from build123d import *

# Parameters (mm, degrees)
F0_W     = 150
F0_H     = 100
F1_DEPTH = 1.5
F2_R     = 1.5
F2_W     = 22.4
F2_H     = 12.1
F3_DEPTH = 3.001
F4_R     = 1.618849898
F4_R_2   = 1.6569654359
F4_R_3   = 1.6400542831
F4_R_4   = 1.6604885459
F5_DEPTH = 3.001


with BuildPart() as f1:
    # F0 (on Top) → F1 (new body, symmetric)
    with BuildSketch(Plane.XY):
        Rectangle(F0_W, F0_H)
    extrude(amount=F1_DEPTH, both=True)

    # F2 (on face) → F3 (cut, through all)
    with BuildSketch(Plane.XY.offset(1.5)):
        with Locations((-55, -30)):
            Circle(F2_R)
        with Locations((-27.3, -30)):
            Circle(F2_R)
        with Locations((-41.15, -30)):
            Rectangle(F2_W, F2_H)
        with Locations((27.3, -30)):
            Circle(F2_R)
        with Locations((55, -30)):
            Circle(F2_R)
        with Locations((41.15, -30)):
            Rectangle(F2_W, F2_H)
        with Locations((27.3, 30)):
            Circle(F2_R)
        with Locations((55, 30)):
            Circle(F2_R)
        with Locations((41.15, 30)):
            Rectangle(F2_W, F2_H)
        with Locations((-55, 30)):
            Circle(F2_R)
        with Locations((-27.3, 30)):
            Circle(F2_R)
        with Locations((-41.15, 30)):
            Rectangle(F2_W, F2_H)
    extrude(amount=-F3_DEPTH, mode=Mode.SUBTRACT)

    # F4 (on face) → F5 (cut, through all)
    with BuildSketch(Plane.XY.offset(1.5)):
        with Locations((-24.7324935626, 26.3731424032)):
            Circle(F4_R)
        with Locations((25.2215412911, 11.3385100679)):
            Circle(F4_R_2)
        with Locations((25.2285262104, -16.3567047299)):
            Circle(F4_R_3)
        with Locations((-25.7276298944, -21.3546585025)):
            Circle(F4_R_4)
    extrude(amount=-F5_DEPTH, mode=Mode.SUBTRACT)


solid = f1.part
Verification items for the finished model (mm, model axes). A direction names the side the tool comes from. Give positions to 0.01 mm unless a question says otherwise; leave off trailing zeros. Order: outer loops, then holes, each group sorted by start corner. A loop starts at its lowest first (then second) coordinate and runs counter-clockwise, first axis right, second up. Notation, with made-up numbers: (-24, -30) -> (-1, -30) arc R22 cw to (-1, -6) -> close; hole circle Ø3 at (87.5, -9.75). An arc over 180 degrees is marked (long way). Answer as CSV lines item,"result".
Q1. Release check for a two-part mould opening along X. For faces 1 (the flat face through (29.95, 30, 0)), 2 (the flat face through (-1, 50, 0)), 3 (the flat face through (-75, -1, 0)) record: +X half, -X half, draft (parallel to the pull), parting line (faces both ways), or undercut.
Solutions:
face 1,"undercut"
face 2,"draft"
face 3,"-X half"
Q2. Sectioned sample at A-A on x = 44.5. Record the cut outline in (y, z), plus the area to 3 significant figures.
Solutions:
outline,"(-50, -1.5) -> (-36.05, -1.5) -> (-36.05, 1.5) -> (-50, 1.5) -> close; (-23.95, -1.5) -> (23.95, -1.5) -> (23.95, 1.5) -> (-23.95, 1.5) -> close; (36.05, -1.5) -> (50, -1.5) -> (50, 1.5) -> (36.05, 1.5) -> close"
area,"227 mm²"
Q3. Scan lines: probe 1 along Y at (x, z) = (-50, -0.85); probe 2 along Y at (x, z) = (-55, -0.4); probe 3 along X at (y, z) = (27, -0.4). Record each from-to range of solid material in increasing order.
Solutions:
probe 1,"y = -50 to -36.05, -23.95 to 23.95, 36.05 to 50"
probe 2,"y = -50 to -31.5, -28.5 to 28.5, 31.5 to 50"
probe 3,"x = -75 to -52.35, -29.95 to -26.23, -23.24 to 29.95, 52.35 to 75"
Q4. Access from +Z, -Z, +X, -X, +Y, -Y to the whole of each face (thin tool, end or side, straight path). Record for faces 4 (the flat face through (-1, 1, -1.5)), 5 (the flat face through (52.35, -30, 0)).
Solutions:
face 4,"-Z, +X, -X, +Y, -Y"
face 5,"+Z, -Z"
Q5. Sectioned sample at C-C on z = -0.1. Count the separate pieces of the cut face and the enclosed holes in it, plus the area to 3 significant figures.
Solutions:
separate pieces,"1"
enclosed holes,"16"
area,"13,800 mm²"
Q6. Sectioned sample at B-B on y = -30. Record the cut outline in (x, z), plus the area to 3 significant figures.
Solutions:
outline,"(-75, -1.5) -> (-56.5, -1.5) -> (-56.5, 1.5) -> (-75, 1.5) -> close; (-53.5, -1.5) -> (-52.35, -1.5) -> (-52.35, 1.5) -> (-53.5, 1.5) -> close; (-29.95, -1.5) -> (-28.8, -1.5) -> (-28.8, 1.5) -> (-29.95, 1.5) -> close; (-25.8, -1.5) -> (25.8, -1.5) -> (25.8, 1.5) -> (-25.8, 1.5) -> close; (28.8, -1.5) -> (29.95, -1.5) -> (29.95, 1.5) -> (28.8, 1.5) -> close; (52.35, -1.5) -> (53.5, -1.5) -> (53.5, 1.5) -> (52.35, 1.5) -> close; (56.5, -1.5) -> (75, -1.5) -> (75, 1.5) -> (56.5, 1.5) -> close"
area,"280 mm²"
